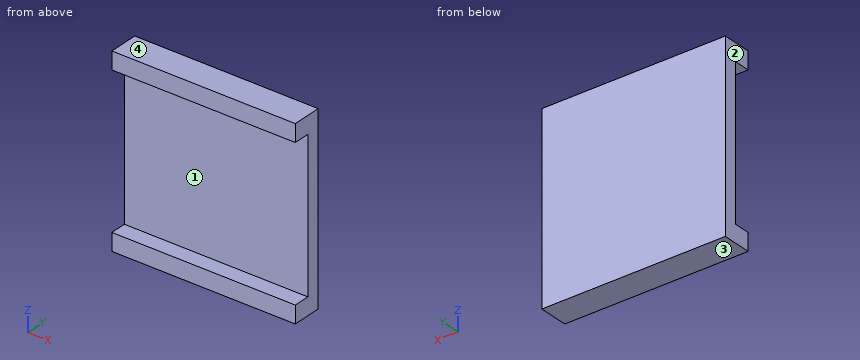
Autodesk Inventor part; units mm, degrees
ref_plane "YZ Plane" through (0, 0, 0) normal (1, 0, 0) x (0, 1, 0)
ref_plane "XZ Plane" through (0, 0, 0) normal (0, 1, 0) x (-1, 0, 0)
ref_plane "XY Plane" through (0, 0, 0) normal (0, 0, 1) x (1, 0, 0)
sketch "Esboço1" plane through (0, 0, 0) normal (0, 1, 0) x (-1, 0, 0)
  line L0 (130.95, 131.25) -> (-130.95, 131.25)
  line L1 (-130.95, 131.25) -> (-130.95, -131.25)
  line L2 (-130.95, -131.25) -> (130.95, -131.25)
  line L3 (130.95, -131.25) -> (130.95, 131.25)
  line L4 (130.95, 131.25) -> (-130.95, -131.25) construction
  line L5 (-130.95, 131.25) -> (130.95, -131.25) construction
  line L6 (130.95, 106.45) -> (-130.95, 106.45)
  line L7 (-130.95, -106.45) -> (130.95, -106.45)
  point P0 (0, 0)
  dimension "d0" = 261.9
  dimension "d1" = 262.5
  dimension "d2" = 24.8
  dimension "d3" = 24.8
extrude "Extrusão1" add sketch "Esboço1" along normal blind 19
extrude "Extrusão2" add sketch "Esboço1" against normal blind 23 contours L3 L6 L1 L0 | L3 L2 L1 L7
properties part number "Tampa"
Geometry check sheet. Reference: the model listing, model coordinates, mm. Face numbers are marked on the shaded views. Give positions to 0.01 mm unless a question says otherwise; leave off trailing zeros. Order: outer loops, then holes, each group sorted by start corner. A loop starts at its lowest first (then second) coordinate and runs counter-clockwise, first axis right, second up. Notation, with made-up numbers: (39.5, 7) - (91.5, 7) arc R8 ccw to (91.5, 22) - close; hole circle Ø4 at (82, -11.75). An arc over 180 degrees is marked (long way). Use one line per item in the form item = value.
1) Sectioned sample at A-A (y = -13.5). Record the boundary of the cut face in (x, z), and give its area (3 significant figures).
Working result:
outline = (-130.95, -131.25) - (130.95, -131.25) - (130.95, -106.45) - (-130.95, -106.45) - close; (-130.95, 106.45) - (130.95, 106.45) - (130.95, 131.25) - (-130.95, 131.25) - close
area = 13,000 mm^2
2) Sectioned sample at B-B (x = 87). Record the boundary of the cut face in (y, z).
Working result:
outline = (-23, -131.25) - (19, -131.25) - (19, 131.25) - (-23, 131.25) - (-23, 106.45) - (0, 106.45) - (0, -106.45) - (-23, -106.45) - close
3) Draft check along Z on the marked faces 1, 2, 3 and 4. Enter one of: released by +Z, released by -Z, zero draft, split by the parting line, or undercut.
Working result:
face_1 = undercut
face_2 = zero draft
face_3 = released by -Z
face_4 = released by +Z
4) Sectioned sample at C-C (z = 93.5). Record the boundary of the cut face in (x, y).
Working result:
outline = (-130.95, 0) - (130.95, 0) - (130.95, 19) - (-130.95, 19) - close
5) Depth check by flat-ended pin: pin 1 Ø3 at (x, z) = (67.5, -7.5) entering from -Y. Enter the tip coordinate at first touch or a pass-through.
Working result:
pin_1 = 0
6) Material ranges on probe 1 along Z at (x, y) = (81, -17); probe 2 along Y at (x, z) = (-105, 46.5), recorded low to high. Write a range as from..to.
Working result:
probe_1 = -131.25..-106.45, 106.45..131.25
probe_2 = 0..19
